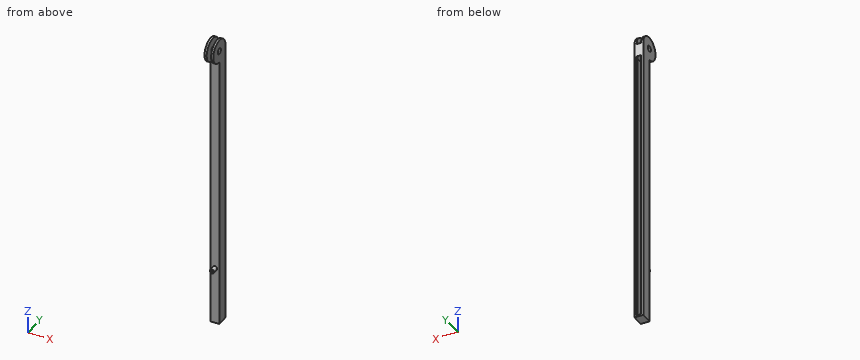
```python
from build123d import *

# Parameters (mm, degrees)
SKETCH1_W           = 60
SKETCH1_H           = 2000
BOSS_EXTRUDE1_DEPTH = 80
CUT_EXTRUDE1_START  = -90
CUT_EXTRUDE1_DEPTH  = 1900
SKETCH3_R           = 80
BOSS_EXTRUDE2_DEPTH = 60
CUT_EXTRUDE2_START  = -15
SKETCH3_2_R         = 80
CUT_EXTRUDE2_DEPTH  = 30
CUT_EXTRUDE3_REACH  = 2004.498
SKETCH4_R           = 20
SKETCH5_R           = 15
SKETCH5_R_2         = 7.5
BOSS_EXTRUDE3_DEPTH = 40
CUT_EXTRUDE4_START  = -15
SKETCH6_R           = 10.5
CUT_EXTRUDE4_DEPTH  = 2


with BuildPart() as part:
    # Sketch1 → Boss-Extrude1 (new body)
    with BuildSketch(Plane(origin=(0, 0, 0), x_dir=(1, 0, 0), z_dir=(0, 1, 0))):
        with Locations((30, 1000)):
            Rectangle(SKETCH1_W, SKETCH1_H)
    extrude(amount=BOSS_EXTRUDE1_DEPTH)

    # Sketch2 → Cut-Extrude1 (cut)
    with BuildSketch(Plane.XY.offset(CUT_EXTRUDE1_START)):
        Polygon((15, 80), (15, 70), (8, 70), (8, 10), (52, 10), (52, 70), (45, 70), (45, 80), align=None)
    extrude(amount=-CUT_EXTRUDE1_DEPTH, mode=Mode.SUBTRACT)

    # Sketch3 → Boss-Extrude2 (add)
    with BuildSketch(Plane(origin=(60, 0, 0), x_dir=(0, 0, -1), z_dir=(1, 0, 0))):
        Circle(SKETCH3_R)
    extrude(amount=-BOSS_EXTRUDE2_DEPTH)

    # Sketch3<2> → Cut-Extrude2 (cut)
    with BuildSketch(Plane(origin=(60, 0, 0), x_dir=(0, 0, -1), z_dir=(1, 0, 0)).offset(CUT_EXTRUDE2_START)):
        Circle(SKETCH3_2_R)
    extrude(amount=-CUT_EXTRUDE2_DEPTH, mode=Mode.SUBTRACT)

    # Cut-Extrude3: up to this face of the body (flat: up to its plane)
    cut_extrude3_end = Plane(part.part.faces().sort_by_distance((0, 35.579997564, -912.895006003))[0])
    # Sketch4 → Cut-Extrude3 (cut, up to the picked face)
    with BuildSketch(Plane(origin=(60, 0, 0), x_dir=(0, 0, -1), z_dir=(1, 0, 0)), mode=Mode.PRIVATE) as cut_extrude3_sk1:
        Circle(SKETCH4_R)
    cut_extrude3_tool1 = split(extrude(cut_extrude3_sk1.sketch, amount=-CUT_EXTRUDE3_REACH, mode=Mode.PRIVATE), bisect_by=cut_extrude3_end, keep=Keep.BOTH, mode=Mode.PRIVATE)
    add(cut_extrude3_tool1.solids().sort_by(Axis((60, 0, 0), (-1, 0, 0)))[0], mode=Mode.SUBTRACT)

    # Sketch5 → Boss-Extrude3 (add)
    with BuildSketch(Plane.XZ):
        with Locations(Location((30, -1600, 0), (0, 0, 90))):
            Circle(SKETCH5_R)
        with Locations(Location((30, -1600, 0), (0, 0, 270))):
            Circle(SKETCH5_R_2, mode=Mode.SUBTRACT)
    extrude(amount=BOSS_EXTRUDE3_DEPTH)

    # Sketch6 → Cut-Extrude4 (cut)
    with BuildSketch(Plane.XZ.offset(40).offset(CUT_EXTRUDE4_START)):
        with Locations(Location((30, -1600, 0), (0, 0, 270))):
            Circle(SKETCH6_R)
    extrude(amount=-CUT_EXTRUDE4_DEPTH, mode=Mode.SUBTRACT)


solid = part.part
```
Geometry check sheet. Reference: the model listing, model coordinates, mm. Coordinates: 2 decimals unless noted, no trailing zeros. Write each loop counter-clockwise with the first axis right and the second up, starting at its lowest first coordinate (ties: lowest second). Pieces come first, ordered by that corner, then holes. Notation, with made-up numbers: M -11.75,27.5 L 25.25,27.5 A30 cw 25.25,59.5 Z; hole C -39.75,-37.5 d3. An arc over 180 degrees is marked long. Use one line per item in the form item = value. Start each with the question number.
1) Go/stop test with flat-tipped pins: pin 1 Ø16.5 at (x, z) = (30, -1599.5) entering from -Y; pin 2 Ø5.5 at (x, z) = (10.5, -1256.5) entering from -Y; pin 3 Ø12 at (x, z) = (30, -1600) entering from +Y; pin 4 Ø10 at (y, z) = (35.5, -1414) entering from -X. Record where each tip stops, or that it passes through.
2) Section check A-A on y = 42. Enter the section's corners in (x, z).
3) Thickness scan on probe 1 along Y at (x, z) = (12.25, 0); probe 2 along Y at (x, z) = (11, -311); probe 3 along X at (y, z) = (58.5, -219). Record the ranges inside material, lowest first. Write a range as from..to.
4) Section check B-B on z = -754.5. Enter the section's corners in (x, y), and give its area (3 significant figures).
Responses:
q1.pin_1 = -40
q1.pin_2 = 0
q1.pin_3 = 10
q1.pin_4 = 0
q2.outline = M 0,-2000 L 60,-2000 L 60,68.09 L 45,68.09 L 45,-68.09 L 15,-68.09 L 15,68.09 L 0,68.09 Z; hole M 8,-1990 L 52,-1990 L 52,-90 L 8,-90 Z
q3.probe_1 = -80..-20, 20..80
q3.probe_2 = 0..10, 70..80
q3.probe_3 = 0..8, 52..60
q4.outline = M 0,0 L 60,0 L 60,80 L 45,80 L 45,70 L 52,70 L 52,10 L 8,10 L 8,70 L 15,70 L 15,80 L 0,80 Z
q4.area = 1,860 mm2
